Could you check a few things on this model? Use its own coordinates, in mm. A direction names the side the tool comes from. Give positions to 0.01 mm unless a question says otherwise; leave off trailing zeros. Order: outer loops, then holes, each group sorted by start corner. A loop starts at its lowest first (then second) coordinate and runs counter-clockwise, first axis right, second up. Notation, with made-up numbers: (-34, 51.5) - (-17, 51.5) arc R16 cw to (-17, 58.5) - close; hole circle Ø9 at (-3.75, -30.75). An arc over 180 degrees is marked (long way). Put each result on its own line as item: value.
from build123d import *

# Parameters (mm, degrees)
F1_R     = 67.5
F1_R_2   = 52.5
F2_DEPTH = 20
F3_R     = 14
F4_DEPTH = 20
F5_W     = 10
F5_H     = 39.4233031694
F6_DEPTH = 20


with BuildPart() as f2:
    # F1 (on Top) → F2 (new body)
    with BuildSketch(Plane.XY):
        Circle(F1_R)
        Circle(F1_R_2, mode=Mode.SUBTRACT)
    extrude(amount=F2_DEPTH)



with BuildPart() as f4:
    # F3 (on Top) → F4 (new body)
    with BuildSketch(Plane.XY):
        Circle(F3_R)
    extrude(amount=F4_DEPTH)


with BuildPart() as f2_1:
    add(f2.part)

    add(f4.part)  # F6 merges F4
    # F5 (on Top) → F6 (join)
    with BuildSketch(Plane.XY):
        with Locations((0, 32.7883484153)):
            Rectangle(F5_W, F5_H)
    extrude(amount=F6_DEPTH)


solid = f2_1.part
1) Suppose I cut it at B-B, the plane y = 0. List the corners of the cut face in (x, z) for me, and give its area (3 significant figures).
Filled in:
outline: (-67.5, 0) - (-52.5, 0) - (-52.5, 20) - (-67.5, 20) - close; (-14, 0) - (14, 0) - (14, 20) - (-14, 20) - close; (52.5, 0) - (67.5, 0) - (67.5, 20) - (52.5, 20) - close
area: 1,160 mm^2
2) Suppose I cut it at D-D, the plane y = -36. List the corners of the cut face in (x, z) for me.
Filled in:
outline: (-57.1, 0) - (-38.21, 0) - (-38.21, 20) - (-57.1, 20) - close; (38.21, 0) - (57.1, 0) - (57.1, 20) - (38.21, 20) - close
3) If I drill on line 1 (X direction, y = 26.5, z = 4.5); line 2 (X direction, y = 46, z = 3); line 3 (Y direction, x = -8, z = 1.25), over which ranges is the centre line in solid material (lowest first)? Write a range as [from, to].
Filled in:
line 1: x = [-62.08, -45.32], [-5, 5], [45.32, 62.08]
line 2: x = [-49.4, -25.3], [-5, 5], [25.3, 49.4]
line 3: y = [-67.02, -51.89], [-11.49, 11.49], [51.89, 67.02]
4) Suppose I cut it at C-C, the plane z = 2.25. List the corners of the cut face in (x, y) for me, and give its area (3 significant figures).
Filled in:
outline: circle Ø135 at (0, 0); hole (-5, 13.08) - (-5, 52.26) arc R52.5 ccw (long way) to (5, 52.26) - (5, 13.08) arc R14 cw (long way) to start
area: 6,660 mm^2
5) Suppose I cut it at A-A, the plane x = 0. List the corners of the cut face in (y, z) for me.
Filled in:
outline: (-67.5, 0) - (-52.5, 0) - (-52.5, 20) - (-67.5, 20) - close; (-14, 0) - (67.5, 0) - (67.5, 20) - (-14, 20) - close
6) We'd pull the mould along X, two halves only. Please class faces 3 (the cylindrical face through (-2.238, -52.452, 9.86)), 4 (the flat face through (-1, 1, 20)), 5 (the cylindrical face through (-53.57, -41.07, 9.86)), 6 (the flat face through (5, 32, 10)): pulls with the +X half, pulls with the -X half, needs draft (parallel to the pull), parting line crosses it, or undercut.
Filled in:
face 3: undercut
face 4: needs draft
face 5: parting line crosses it
face 6: undercut
7) Which directions (+Z, -Z, +X, -X, +Y, -Y) give clear straight access to the entire face, cutting with the end or side of a thin tool? Please do faces 1 (the flat face through (-5, 32, 10)), 2 (the flat face through (-1, 1, 0)).
Filled in:
face 1: +Z, -Z
face 2: -Z, +X, -X, +Y, -Y
8) I'm going to push flat-ended pins straight in: pin 1 (8 mm diameter, centred on y = -36.5, z = 18, fed in from +X); pin 2 (12 mm diameter, centred on y = -21.5, z = 12, fed in from +X); pin 3 (10 mm diameter, centred on y = 39, z = 12.5, fed in from +X). Where does each tip first touch, or does it pass through?
Filled in:
pin 1: stops at x = 59.16
pin 2: stops at x = 65.7
pin 3: stops at x = 58.31
